Can you work these out from the model? Positions are in its coordinate system, mm. Give positions to 0.01 mm unless a question says otherwise; leave off trailing zeros. Write each loop counter-clockwise with the first axis right and the second up, starting at its lowest first coordinate (ties: lowest second). Pieces come first, ordered by that corner, then holes. Notation, with made-up numbers: (-10, 59.5) -> (15, 59.5) arc R26 ccw to (15, 92.5) -> close; hole circle Ø11 at (-14, 49). An arc over 180 degrees is marked (long way). One line per item, written item: value.
from build123d import *

# Parameters (mm, degrees)
SKETCH22_W                      = 3.9
SKETCH22_H                      = 3.9
F_40_SERIES_TS40_120LM_1_DEPTH  = 260
M8X1_25_TAPPED_HOLE1_AT_2_COUNT = 2
M8X1_25_TAPPED_HOLE1_AT_2_PITCH = 40


with BuildPart() as part:
    # Sketch22 → 40 series TS40-120LM(1) (new body)
    with BuildSketch(Plane(origin=(0, 0, 130), x_dir=(-1, 0, 0), z_dir=(0, 0, -1))):
        with BuildLine():
            Line((15.3, -35.9), (20, -35.9))
            Line((20, -35.9), (20, -4.1))
            Line((20, -4.1), (15.3, -4.1))
            Line((15.3, -4.1), (15.3, -7.6))
            Line((15.3, -7.6), (17.65, -7.6))
            Line((17.65, -7.6), (17.65, -10.1))
            Line((17.65, -10.1), (13.6, -10.1))
            Line((13.6, -10.1), (7.6, -4.1))
            Line((7.6, -4.1), (7.6, 4.1))
            Line((7.6, 4.1), (13.6, 10.1))
            Line((13.6, 10.1), (17.65, 10.1))
            Line((17.65, 10.1), (17.65, 7.6))
            Line((17.65, 7.6), (15.3, 7.6))
            Line((15.3, 7.6), (15.3, 4.1))
            Line((15.3, 4.1), (20, 4.1))
            Line((20, 4.1), (20, 35.9))
            Line((20, 35.9), (15.3, 35.9))
            Line((15.3, 35.9), (15.3, 32.4))
            Line((15.3, 32.4), (17.65, 32.4))
            Line((17.65, 32.4), (17.65, 29.9))
            Line((17.65, 29.9), (13.6, 29.9))
            Line((13.6, 29.9), (7.6, 35.9))
            Line((7.6, 35.9), (7.6, 44.1))
            Line((7.6, 44.1), (13.6, 50.1))
            Line((13.6, 50.1), (17.65, 50.1))
            Line((17.65, 50.1), (17.65, 47.6))
            Line((17.65, 47.6), (15.3, 47.6))
            Line((15.3, 47.6), (15.3, 44.1))
            Line((15.3, 44.1), (20, 44.1))
            Line((20, 44.1), (20, 57.5))
            ThreePointArc((20, 57.5), (19.267766953, 59.267766953), (17.5, 60))
            Line((17.5, 60), (4.1, 60))
            Line((4.1, 60), (4.1, 55.3))
            Line((4.1, 55.3), (7.6, 55.3))
            Line((7.6, 55.3), (7.6, 57.65))
            Line((7.6, 57.65), (10.1, 57.65))
            Line((10.1, 57.65), (10.1, 53.6))
            Line((10.1, 53.6), (4.1, 47.6))
            Line((4.1, 47.6), (-4.1, 47.6))
            Line((-4.1, 47.6), (-10.1, 53.6))
            Line((-10.1, 53.6), (-10.1, 57.65))
            Line((-10.1, 57.65), (-7.6, 57.65))
            Line((-7.6, 57.65), (-7.6, 55.3))
            Line((-7.6, 55.3), (-4.1, 55.3))
            Line((-4.1, 55.3), (-4.1, 60))
            Line((-4.1, 60), (-17.5, 60))
            ThreePointArc((-17.5, 60), (-19.267766953, 59.267766953), (-20, 57.5))
            Line((-20, 57.5), (-20, 44.1))
            Line((-20, 44.1), (-15.3, 44.1))
            Line((-15.3, 44.1), (-15.3, 47.6))
            Line((-15.3, 47.6), (-17.65, 47.6))
            Line((-17.65, 47.6), (-17.65, 50.1))
            Line((-17.65, 50.1), (-13.6, 50.1))
            Line((-13.6, 50.1), (-7.6, 44.1))
            Line((-7.6, 44.1), (-7.6, 35.9))
            Line((-7.6, 35.9), (-13.6, 29.9))
            Line((-13.6, 29.9), (-17.65, 29.9))
            Line((-17.65, 29.9), (-17.65, 32.4))
            Line((-17.65, 32.4), (-15.3, 32.4))
            Line((-15.3, 32.4), (-15.3, 35.9))
            Line((-15.3, 35.9), (-20, 35.9))
            Line((-20, 35.9), (-20, 4.1))
            Line((-20, 4.1), (-15.3, 4.1))
            Line((-15.3, 4.1), (-15.3, 7.6))
            Line((-15.3, 7.6), (-17.65, 7.6))
            Line((-17.65, 7.6), (-17.65, 10.1))
            Line((-17.65, 10.1), (-13.6, 10.1))
            Line((-13.6, 10.1), (-7.6, 4.1))
            Line((-7.6, 4.1), (-7.6, -4.1))
            Line((-7.6, -4.1), (-13.6, -10.1))
            Line((-13.6, -10.1), (-17.65, -10.1))
            Line((-17.65, -10.1), (-17.65, -7.6))
            Line((-17.65, -7.6), (-15.3, -7.6))
            Line((-15.3, -7.6), (-15.3, -4.1))
            Line((-15.3, -4.1), (-20, -4.1))
            Line((-20, -4.1), (-20, -35.9))
            Line((-20, -35.9), (-15.3, -35.9))
            Line((-15.3, -35.9), (-15.3, -32.4))
            Line((-15.3, -32.4), (-17.65, -32.4))
            Line((-17.65, -32.4), (-17.65, -29.9))
            Line((-17.65, -29.9), (-13.6, -29.9))
            Line((-13.6, -29.9), (-7.6, -35.9))
            Line((-7.6, -35.9), (-7.6, -44.1))
            Line((-7.6, -44.1), (-13.6, -50.1))
            Line((-13.6, -50.1), (-17.65, -50.1))
            Line((-17.65, -50.1), (-17.65, -47.6))
            Line((-17.65, -47.6), (-15.3, -47.6))
            Line((-15.3, -47.6), (-15.3, -44.1))
            Line((-15.3, -44.1), (-20, -44.1))
            Line((-20, -44.1), (-20, -57.5))
            ThreePointArc((-20, -57.5), (-19.267766953, -59.267766953), (-17.5, -60))
            Line((-17.5, -60), (-4.1, -60))
            Line((-4.1, -60), (-4.1, -55.3))
            Line((-4.1, -55.3), (-7.6, -55.3))
            Line((-7.6, -55.3), (-7.6, -57.65))
            Line((-7.6, -57.65), (-10.1, -57.65))
            Line((-10.1, -57.65), (-10.1, -53.6))
            Line((-10.1, -53.6), (-4.1, -47.6))
            Line((-4.1, -47.6), (4.1, -47.6))
            Line((4.1, -47.6), (10.1, -53.6))
            Line((10.1, -53.6), (10.1, -57.65))
            Line((10.1, -57.65), (7.6, -57.65))
            Line((7.6, -57.65), (7.6, -55.3))
            Line((7.6, -55.3), (4.1, -55.3))
            Line((4.1, -55.3), (4.1, -60))
            Line((4.1, -60), (17.5, -60))
            ThreePointArc((17.5, -60), (19.267766953, -59.267766953), (20, -57.5))
            Line((20, -57.5), (20, -44.1))
            Line((20, -44.1), (15.3, -44.1))
            Line((15.3, -44.1), (15.3, -47.6))
            Line((15.3, -47.6), (17.65, -47.6))
            Line((17.65, -47.6), (17.65, -50.1))
            Line((17.65, -50.1), (13.6, -50.1))
            Line((13.6, -50.1), (7.6, -44.1))
            Line((7.6, -44.1), (7.6, -35.9))
            Line((7.6, -35.9), (13.6, -29.9))
            Line((13.6, -29.9), (17.65, -29.9))
            Line((17.65, -29.9), (17.65, -32.4))
            Line((17.65, -32.4), (15.3, -32.4))
            Line((15.3, -32.4), (15.3, -35.9))
        make_face()
        Polygon((-4.1, -7.6), (4.1, -7.6), (8.6, -12.1), (17.65, -12.1), (17.65, -27.9), (8.6, -27.9), (4.1, -32.4), (-4.1, -32.4), (-8.6, -27.9), (-17.65, -27.9), (-17.65, -12.1), (-8.6, -12.1), align=None, mode=Mode.SUBTRACT)
        Polygon((-4.1, 7.6), (-8.6, 12.1), (-17.65, 12.1), (-17.65, 27.9), (-8.6, 27.9), (-4.1, 32.4), (4.1, 32.4), (8.6, 27.9), (17.65, 27.9), (17.65, 12.1), (8.6, 12.1), (4.1, 7.6), align=None, mode=Mode.SUBTRACT)
        with Locations((15.55, -55.55)):
            Rectangle(SKETCH22_W, SKETCH22_H, mode=Mode.SUBTRACT)
        with Locations((-15.55, -55.55)):
            Rectangle(SKETCH22_W, SKETCH22_H, mode=Mode.SUBTRACT)
        with Locations((-15.55, 55.55)):
            Rectangle(SKETCH22_W, SKETCH22_H, mode=Mode.SUBTRACT)
        with Locations((15.55, 55.55)):
            Rectangle(SKETCH22_W, SKETCH22_H, mode=Mode.SUBTRACT)
        with BuildLine():
            ThreePointArc((0, -43.35), (3.35, -40), (0, -36.65))
            ThreePointArc((0, -36.65), (-3.35, -40), (0, -43.35))
        make_face(mode=Mode.SUBTRACT)
        with BuildLine():
            ThreePointArc((3.35, 0), (0, -3.35), (-3.35, 0))
            ThreePointArc((-3.35, 0), (0, 3.35), (3.35, 0))
        make_face(mode=Mode.SUBTRACT)
        with BuildLine():
            ThreePointArc((0, 43.35), (-3.35, 40), (0, 36.65))
            ThreePointArc((0, 36.65), (3.35, 40), (0, 43.35))
        make_face(mode=Mode.SUBTRACT)
    extrude(amount=F_40_SERIES_TS40_120LM_1_DEPTH)

    # Sketch4 → M8x1.25 Tapped Hole1 (revolve, cut)
    with BuildSketch(Plane(origin=(0, 0, 130), x_dir=(0, -1, 0), z_dir=(1, 0, 0))):
        Polygon((0, 0), (0, 32.042926105), (3.4, 30), (3.4, 0), align=None)
    m8x1_25_tapped_hole1 = revolve(axis=Axis((0, 0, 136.35), (0, 0, -1)), mode=Mode.SUBTRACT)

    # M8x1.25 Tapped Hole1 at 2: M8x1.25 Tapped Hole1 ×2
    with Locations(*[(0, i * M8X1_25_TAPPED_HOLE1_AT_2_PITCH, 0) for i in range(1, M8X1_25_TAPPED_HOLE1_AT_2_COUNT)]):
        add(m8x1_25_tapped_hole1, mode=Mode.SUBTRACT)

    # Mirror1: M8x1.25 Tapped Hole1 across plane
    add(m8x1_25_tapped_hole1.mirror(Plane.XY), mode=Mode.SUBTRACT)

    # Mirror1 copy 1 sketch → Mirror1 copy 1 (revolve, cut)
    with BuildSketch(Plane(origin=(0, 40, -130), x_dir=(0, -1, 0), z_dir=(1, 0, 0))):
        Polygon((0, 0), (0, -32.042926105), (3.4, -30), (3.4, 0), align=None)
    revolve(axis=Axis((0, 40, -136.35), (0, 0, -1)), mode=Mode.SUBTRACT)


solid = part.part
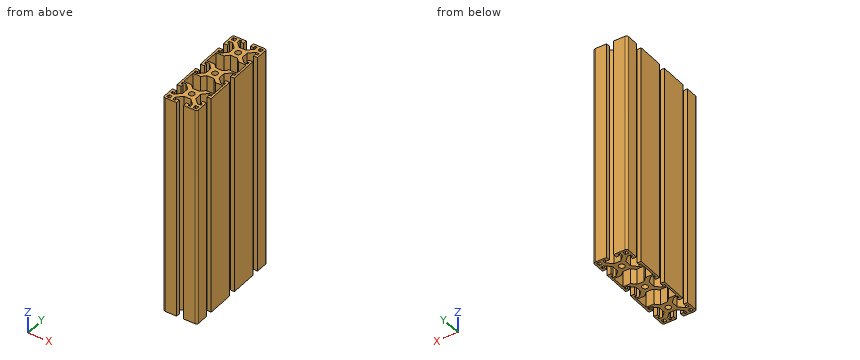
1) If we section it at B-B (y = 40): Write out the boundary of the cut face in (x, z).
Answer list:
outline: (-7.6, -130) -> (-3.4, -130) -> (-3.4, -100) -> (-3.35, -99.97) -> (-3.35, 99.97) -> (-3.4, 100) -> (-3.4, 130) -> (-7.6, 130) -> close; (3.35, -99.97) -> (3.4, -100) -> (3.4, -130) -> (7.6, -130) -> (7.6, 130) -> (3.4, 130) -> (3.4, 100) -> (3.35, 99.97) -> close
2) If we section it at A-A (y = 21): Write out the boundary of the cut face in (x, z).
Answer list:
outline: (-20, -130) -> (-17.65, -130) -> (-17.65, 130) -> (-20, 130) -> close; (17.65, -130) -> (20, -130) -> (20, 130) -> (17.65, 130) -> close
3) Will these pins go through, and if not, where does the flat tip stop? pin 1 (4 mm diameter, centred on y = -0.5, z = -14.5, fed in from +X); pin 2 (2 mm diameter, centred on y = 2.5, z = 100.5, fed in from -X).
Answer list:
pin 1: stops at x = 7.6
pin 2: stops at x = -7.6
4) If we section it at C-C (z = -78): State how many separate pieces and enclosed holes the cut face has, and give its area (3 significant figures).
Answer list:
separate pieces: 1
enclosed holes: 9
area: 1,930 mm^2
5) I need wall thicknesses on L1, parallel to Y at x = -0.5, z = 35; L2, parallel to Y at x = -3.5, z = -10.5; L3, parallel to X at y = 40, z = -112.5. Which ranges of each line are inside material? Lowest first, please.
Answer list:
L1: y = -47.6 to -43.31, -36.69 to -32.4, -7.6 to -3.31, 3.31 to 7.6, 32.4 to 36.69, 43.31 to 47.6
L2: y = -47.6 to -32.4, -7.6 to 7.6, 32.4 to 47.6
L3: x = -7.6 to -3.4, 3.4 to 7.6
